CAD build for the part. Positions are in the model's coordinates, mm. A direction names the side the tool comes from. Give positions to 0.01 mm unless a question says otherwise; leave off trailing zeros. Order: outer loops, then holes, each group sorted by start corner. A loop starts at its lowest first (then second) coordinate and runs counter-clockwise, first axis right, second up. Notation, with made-up numbers: (22, 57.5) -> (29, 57.5) arc R25 ccw to (29, 88.5) -> close; hole circle Ø3 at (0, 82). An arc over 180 degrees is marked (long way). Use one line per item in the form item = value. Start each with the question number.
1) Drop flat-ended pins along their axis: P1, Ø14.5, axis at x = -37.79, y = 8.86, coming from the -Z side; P2, Ø2, axis at y = -5, z = -3, coming from the +X side. Give the stop position or say it passes through.
2) Mould opens along Y. For faces 3 (the face through (-14, 31.886, -13)), 4 (the face through (-15, -24.8, -13)), 5 (the face through (1, -11.219, -13)) say: pulls with the +Y half, pulls with the -Y half, needs draft (parallel to the pull), parting line crosses it, or undercut.
3) Cut at A-A, the plane x = -3.5. Give the cut face in (y, z), and give its area (3 significant figures).
4) Cut at C-C, the plane z = -16.25. Give the cut face in (x, y).
5) Probe line 1 (Y direction, x = -10, z = -19.5); line 2 (X direction, y = -1.5, z = -2.5); line 3 (X direction, y = 16.5, z = -13.5). List the from-to ranges inside material, lowest first.
6) Cut at B-B, the plane y = 5. Give the cut face in (x, z), and give its area (3 significant figures).
7) Tool access for faces 1 (the face through (0, 10.629, -13)), 2 (the face through (-24, 4, 0)): list every direction of +Z, -Z, +X, -X, +Y, -Y with a clear straight run to the whole face (end or side of a thin tool).
from build123d import *

# Parameters (mm, degrees)
F0_R     = 9.152436
F1_DEPTH = 25.4


with BuildPart() as f1:
    # F0 (on Top) → F1 (new body)
    with BuildSketch(Plane.XY):
        Polygon((21.552509, 31.885903), (-51.371735, 31.885903), (-51.371735, -24.800148), (21.552509, -24.800148), (21.552509, -11.219114), (-20.96203, -11.219114), (-20.96203, 10.628635), (21.552509, 10.628635), align=None)
        with Locations((-37.790701, 8.857195)):
            Circle(F0_R, mode=Mode.SUBTRACT)
    extrude(amount=-F1_DEPTH)


solid = f1.part
Result:
q1.P1 = through
q1.P2 = -20.96
q2.face_3 = pulls with the +Y half
q2.face_4 = pulls with the -Y half
q2.face_5 = undercut
q3.outline = (-24.8, -25.4) -> (-11.22, -25.4) -> (-11.22, 0) -> (-24.8, 0) -> close; (10.63, -25.4) -> (31.89, -25.4) -> (31.89, 0) -> (10.63, 0) -> close
q3.area = 885 mm²
q4.outline = (-51.37, -24.8) -> (21.55, -24.8) -> (21.55, -11.22) -> (-20.96, -11.22) -> (-20.96, 10.63) -> (21.55, 10.63) -> (21.55, 31.89) -> (-51.37, 31.89) -> close; hole circle Ø18.3 at (-37.79, 8.86)
q5.line_1 = -24.8 to -11.22, 10.63 to 31.89
q5.line_2 = -51.37 to -20.96
q5.line_3 = -51.37 to -42.83, -32.76 to 21.55
q6.outline = (-51.37, -25.4) -> (-46.09, -25.4) -> (-46.09, 0) -> (-51.37, 0) -> close; (-29.49, -25.4) -> (-20.96, -25.4) -> (-20.96, 0) -> (-29.49, 0) -> close
q6.area = 351 mm²
q7.face_1 = +Z, -Z, +X
q7.face_2 = +Z, +X, -X, +Y, -Y
